Geometry: final body of the model. Coordinates: model frame, mm. Face numbers are marked on the shaded views. A direction names the side the tool comes from. Give positions to 0.01 mm unless a question says otherwise; leave off trailing zeros. Write each loop counter-clockwise with the first axis right and the second up, starting at its lowest first coordinate (ties: lowest second). Pieces come first, ordered by that corner, then holes.
Q1. Pin query (flat end, axial travel): pin 1 Ø3 at (x, z) = (3.5, 12.5) entering from +Y; pin 2 Ø6 at (y, z) = (-1, 7) entering from +X; pin 3 Ø1.5 at (y, z) = (3, 3) entering from +X. Return the tip coordinate at first contact, or that it passes through.
Q2. Section A-A (z = 5.5). Return the cut outline in (x, y) (3 decimals).
Q3. Reachability of the marked faces 1 and 2 from +Z, -Z, +X, -X, +Y, -Y: full face, straight path, thin tool, end or side. Return the list, or none.
Q4. Line query: line 1 (X direction, y = 10.5, z = 3.75); line 2 (Z direction, x = -14, y = 8); line 3 (X direction, y = 6.5, z = 9.5). Output: solid intervals per line, ascending.
Q5. Mould query, pull axis X, two halves, no side actions, for the marked faces 3, 4, 5 and 6. Classes: +X half, -X half, draft (parallel to the pull), parting line (faces both ways), or undercut.
Q6. Section D-D (x = 2.5). Return the cut outline in (y, z), plus the area to 3 significant figures.
Q7. Section C-C (y = 1). Return the cut outline in (x, z), plus the area to 3 significant figures.
Q8. Section B-B (x = -8). Return the cut outline in (y, z).
from build123d import *

# Parameters (mm, degrees)
F0_R     = 3.636094
F1_DEPTH = 14.224
F2_T     = -2.54


with BuildPart() as f1:
    # F0 (on Top) → F1 (new body)
    with BuildSketch(Plane.XY):
        Polygon((-17.40883, -6.778608), (-3.317572, -10.594991), (8.451953, -1.957478), (9.037052, 12.629708), (-2.002867, 22.182119), (-16.354518, 19.506593), (-23.210817, 6.617858), align=None)
        with Locations((-5.8684, 5.959329)):
            Circle(F0_R, mode=Mode.SUBTRACT)
    extrude(amount=F1_DEPTH)

    # F2
    f2_openings = [f1.faces().sort_by_distance(p)[0] for p in [
        (-10.242999, -8.242978, 14.224),
    ]]
    offset(amount=F2_T, openings=f2_openings)


solid = f1.part
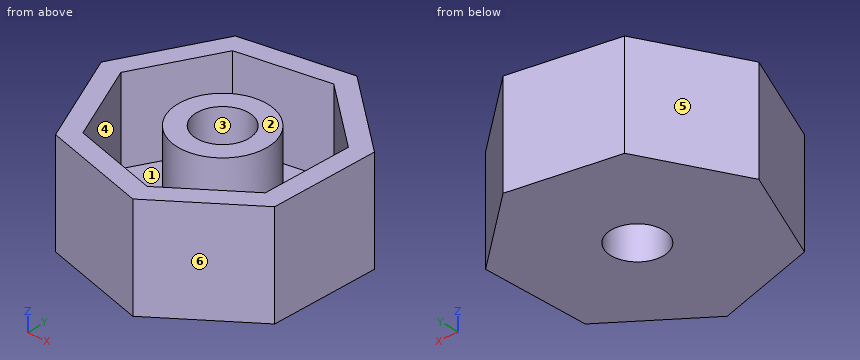
Computed:
1. pin 1: stops at y = 18.72
1. pin 2: stops at x = 8.61
1. pin 3: stops at x = 8.68
2. outline: (-23.211, 6.618) - (-17.409, -6.779) - (-3.318, -10.595) - (8.452, -1.957) - (9.037, 12.63) - (-2.003, 22.182) - (-16.355, 19.507) - close; circle Ø12.352 at (-5.868, 5.959); hole (-20.394, 6.505) - (-15.564, -4.647) - (-3.834, -7.824) - (5.963, -0.633) - (6.45, 11.509) - (-2.74, 19.461) - (-14.687, 17.234) - close; hole circle Ø7.272 at (-5.868, 5.959)
3. face 1: +Z
3. face 2: +Z, +X, -X, +Y, -Y
4. line 1: x = -21.15 to -18.27, -10.05 to -1.68, 6.41 to 8.95
4. line 2: z = 0 to 2.54
4. line 3: x = -23.16 to -20.39, -12.02 to -9.46, -2.27 to 0.28, 6.25 to 8.79
5. face 3: undercut
5. face 4: undercut
5. face 5: -X half
5. face 6: +X half
6. outline: (-6.33, 0) - (18.29, 0) - (18.29, 14.22) - (14.93, 14.22) - (14.93, 2.54) - (-3.17, 2.54) - (-3.17, 14.22) - (-6.33, 14.22) - close
6. area: 139 mm2
7. outline: (-20.78, 0) - (8.57, 0) - (8.57, 14.22) - (6.03, 14.22) - (6.03, 2.54) - (-2.19, 2.54) - (-2.19, 14.22) - (-9.55, 14.22) - (-9.55, 2.54) - (-18.01, 2.54) - (-18.01, 14.22) - (-20.78, 14.22) - close
7. area: 223 mm2
8. outline: (-9.33, 0) - (3.01, 0) - (3.01, 14.22) - (0.16, 14.22) - (0.16, 2.54) - (-6.7, 2.54) - (-6.7, 14.22) - (-9.33, 14.22) - close; (8.91, 0) - (21.06, 0) - (21.06, 14.22) - (18.48, 14.22) - (18.48, 2.54) - (11.76, 2.54) - (11.76, 14.22) - (8.91, 14.22) - close
